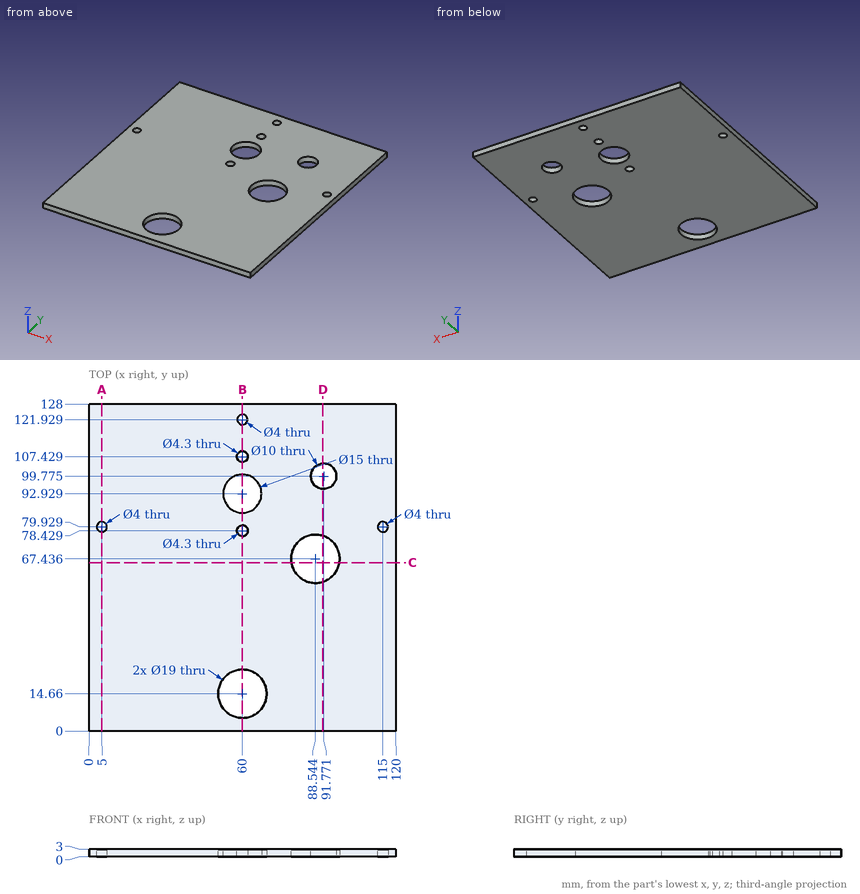
Answer from the drawing. Dimensions are ordinates in mm from the lowest x, y and z of the part. Coordinates: 2 decimals unless noted, no trailing zeros. Write each loop counter-clockwise with the first axis right and the second up, starting at its lowest first coordinate (ties: lowest second). Pieces come first, ordered by that corner, then holes. Notation, with made-up numbers: M -15.5,1.25 L 20.5,1.25 A22 cw 20.5,35.25 Z; hole C -28,87 d10. An arc over 180 degrees is marked long. Put each result on its own line as item: value. Start each with the question number.
1. A cutting plane is placed at A-A on x = 5. Write down the section's boundary in (y, z), then the cut area to 3 significant figures.
2. A cutting plane is placed at B-B on x = 60. Write down the section's boundary in (y, z), then the cut area to 3 significant figures.
3. Consider line 1 (Y direction, x = 60, z = 1.6); line 2 (Y direction, x = 66.5, z = 1.75) (1 decimal); line 3 (X direction, y = 15, z = 1.6). Determine where each line is inside the solid, lowest interval first. Write a range as from..to.
4. A cutting plane is placed at C-C on y = 66. Write down the section's boundary in (x, z) (1 decimal).
5. A flat-ended cylindrical pin translates along its axis: P1, Ø13.5, axis at x = 60, y = 92.93, coming from the -Z side. Find the tip coordinate at first contact, or state that the pin passes through.
6. A cutting plane is placed at D-D on x = 91.5. Write down the section's boundary in (y, z) (1 decimal).
Resolved:
1. outline: M 0,0 L 77.93,0 L 77.93,3 L 0,3 Z; M 81.93,0 L 128,0 L 128,3 L 81.93,3 Z
1. area: 372 mm2
2. outline: M 0,0 L 5.16,0 L 5.16,3 L 0,3 Z; M 24.16,0 L 76.28,0 L 76.28,3 L 24.16,3 Z; M 80.58,0 L 85.43,0 L 85.43,3 L 80.58,3 Z; M 100.43,0 L 105.28,0 L 105.28,3 L 100.43,3 Z; M 109.58,0 L 119.93,0 L 119.93,3 L 109.58,3 Z; M 123.93,0 L 128,0 L 128,3 L 123.93,3 Z
2. area: 244 mm2
3. line 1: y = 0..5.16, 24.16..76.28, 80.58..85.43, 100.43..105.28, 109.58..119.93, 123.93..128
3. line 2: y = 0..7.7, 21.6..89.2, 96.7..128
3. line 3: x = 0..50.51, 69.49..120
4. outline: M 0,0 L 79.2,0 L 79.2,3 L 0,3 Z; M 97.9,0 L 120,0 L 120,3 L 97.9,3 Z
5. P1: passes through
6. outline: M 0,0 L 58.4,0 L 58.4,3 L 0,3 Z; M 76.5,0 L 94.8,0 L 94.8,3 L 76.5,3 Z; M 104.8,0 L 128,0 L 128,3 L 104.8,3 Z
